Work out the finished part from the listing and answer in its coordinate system (mm). Give positions to 0.01 mm unless a question says otherwise; leave off trailing zeros. Loops run counter-clockwise (first coordinate to the right, second up) from the corner with the lowest first, then second, coordinate; pieces in that order, holes last. Notation, with made-up numbers: M 6.25,-1.75 L 12.25,-1.75 A24 cw 12.25,35.25 Z; hole C 80.5,24.5 d2. An arc over 180 degrees is marked long. Write item = value, one per line. Start each with the question number.
1. Section A-A on z = 1.85 is taken. Give the number of separate pieces and of enclosed holes in the cut face, plus the area to 3 significant figures.
2. Section C-C on y = 202.5 is taken. Determine the outline of the cut face in (x, z), plus the area to 4 significant figures.
3. Consider L1, parallel to Y at x = 146.5, z = 2.75; L2, parallel to X at y = 201, z = 3.15; L3, parallel to Y at x = 185, z = 5.05. Determine where each line is inside the solid, lowest interval first. Write a range as [from, to].
4. Section B-B on y = 85 is taken. Determine the outline of the cut face in (x, z), plus the area to 3 significant figures.
5. Flat-ended cylindrical pins translate along their axes: pin 1 Ø3 at (y, z) = (186, 4) entering from -X; pin 2 Ø1.6 at (y, z) = (170, 4) entering from +X. Find the tip coordinate at first contact, or state that the pin passes through.
6. The mould has two halves that part along X. Classify faces 1 (the face through (105, 164, 5.5)), 2 (the face through (64.105, 184.197, 2.788)): released by +X, released by -X, zero draft, split by the parting line, or undercut.
Autodesk Inventor part; units mm, degrees
ref_plane "YZ Plane" through (0, 0, 0) normal (1, 0, 0) x (0, 1, 0)
ref_plane "XZ Plane" through (0, 0, 0) normal (0, 1, 0) x (-1, 0, 0)
ref_plane "XY Plane" through (0, 0, 0) normal (0, 0, 1) x (1, 0, 0)
sketch "Sketch1" plane through (0, 0, 0) normal (0, 0, 1) x (1, 0, 0)
  line L0 (0, 0) -> (106.5, 0)
  line L1 (106.5, 0) -> (106.5, 232.6) construction
  line L2 (106.5, 232.6) -> (0, 232.6)
  line L3 (0, 232.6) -> (0, 0)
  line L4 (213, 0) -> (106.5, 0)
  line L5 (106.5, 232.6) -> (213, 232.6)
  line L6 (213, 232.6) -> (213, 0)
  line L7 (5.5, 100) -> (5.5, 232.599)
  line L8 (5.5, 232.599) -> (0, 232.599)
  line L9 (0, 232.599) -> (0, 100)
  line L10 (0, 100) -> (5.5, 100)
  line L11 (5.5, 100) -> (0, 232.599) construction
  line L12 (5.5, 232.599) -> (0, 100) construction
  line L13 (31, 100) -> (31, 232.599)
  line L14 (31, 232.599) -> (25.5, 232.599)
  line L15 (25.5, 232.599) -> (25.5, 100)
  line L16 (25.5, 100) -> (31, 100)
  line L17 (31, 100) -> (25.5, 232.599) construction
  line L18 (31, 232.599) -> (25.5, 100) construction
  line L19 (96.5, 100) -> (96.5, 232.599)
  line L20 (96.5, 232.599) -> (91.5, 232.599)
  line L21 (91.5, 232.599) -> (91.5, 100)
  line L22 (91.5, 100) -> (96.5, 100)
  line L23 (96.5, 100) -> (91.5, 232.599) construction
  line L24 (96.5, 232.599) -> (91.5, 100) construction
  line L25 (207.5, 100) -> (207.5, 232.599)
  line L26 (207.5, 232.599) -> (213, 232.599)
  line L27 (213, 232.599) -> (213, 100)
  line L28 (213, 100) -> (207.5, 100)
  line L29 (207.5, 100) -> (213, 232.599) construction
  line L30 (207.5, 232.599) -> (213, 100) construction
  line L31 (182, 100) -> (182, 232.599)
  line L32 (182, 232.599) -> (187.5, 232.599)
  line L33 (187.5, 232.599) -> (187.5, 100)
  line L34 (187.5, 100) -> (182, 100)
  line L35 (182, 100) -> (187.5, 232.599) construction
  line L36 (182, 232.599) -> (187.5, 100) construction
  line L37 (116.5, 100) -> (116.5, 232.599)
  line L38 (116.5, 232.599) -> (121.5, 232.599)
  line L39 (121.5, 232.599) -> (121.5, 100)
  line L40 (121.5, 100) -> (116.5, 100)
  line L41 (116.5, 100) -> (121.5, 232.599) construction
  line L42 (116.5, 232.599) -> (121.5, 100) construction
  line L43 (2.75, 166.2995) -> (94, 166.2995) construction
  point P0 (28.25, 166.2995)
  point P1 (210.25, 166.2995)
  point P2 (184.75, 166.2995)
  point P3 (119, 166.2995)
  point P4 (0, 100)
  point P5 (213, 100)
  point P6 (0, 232.599)
  dimension "d0" = 232.6
  dimension "d1" = 106.5
  dimension "d4" = 5.5
  dimension "d6" = 5.5
  dimension "d8" = 5
  dimension "d10" = 10
  dimension "d11" = 20
  dimension "d12" = 0
  dimension "d19" = 100
  dimension "d20" = 0.001
extrude "Extrusion1" add sketch "Sketch1" along normal blind 5.5 contours L3 L10 L7 L2 L15 L16 L13 L21 L22 L19 L5 L37 L40 L39 L31 L34 L33 L25 L28 L6 L4 L0
ref_plane "Work Plane3" through (61.25, 100, 0) normal (1, 0, 0) x (0, 0, -1)
sketch "Sketch2" plane through (0, 0, 5.5) normal (0, 0, 1) x (1, 0, 0)
  line L0 (0, 232.6) -> (213, 232.6)
  line L1 (213, 232.6) -> (213, 322.6)
  line L2 (213, 322.6) -> (0, 322.6)
  line L3 (0, 322.6) -> (0, 232.6)
  line L4 (213, 232.599) -> (213, 232.6)
  point P0 (0, 0)
  dimension "d15" = 90
extrude "Extrusion2" add sketch "Sketch2" against normal blind 5.5
sketch "Sketch3" plane through (0, 0, 5.5) normal (0, 0, 1) x (1, 0, 0)
  line L0 (213, 322.6) -> (0, 322.6) construction
  line L1 (31, 232.599) -> (31, 100) construction
  line L2 (91.5, 100) -> (91.5, 232.599) construction
  line L3 (121.5, 232.599) -> (121.5, 100) construction
  line L4 (31, 166.2995) -> (91.5, 166.2995) construction
  line L5 (91.5, 166.2995) -> (121.5, 166.2995) construction
  line L6 (106.5, 166.2995) -> (106.5, 322.6) construction
  circle A0 centre (66.5, 182) radius 3.25
  circle A1 centre (66.5, 85) radius 3.25
  circle A2 centre (146.5, 182) radius 3.25
  circle A3 centre (146.5, 85) radius 3.25
  line L7 (66.5, 85) -> (66.5, 182) construction
  line L8 (0, 0) -> (213, 0)
  dimension "d21" = 6.5
  dimension "d23" = 97
  dimension "d28" = 40
  dimension "d29" = 85
extrude "Extrusion3" cut sketch "Sketch3" against normal blind 10
ref_plane "Work Plane4" through (106.5, 100, 0) normal (1, 0, 0) x (0, 0, -1)
equation "\"d0\" = sidewallL + Uthick"
equation "\"d10\" = 0.5 * midbottomw"
equation "\"d11\" = lrbottomw"
equation "\"d19\" = Uthick"
equation "\"d15\" = wireL"
equation "\"d28\" = 0.5 * marshdistance"
equation "\"thick\" = 0.5"
equation "\"lrlr\" = 19"
equation "\"lrmid\" = 19.9"
equation "\"lrdepth\" = 3.3"
equation "\"mlr\" = 16.6"
equation "\"mmid\" = 24.7"
equation "\"mdepth\" = 4.5"
equation "\"lrltotal\" = 126.6"
equation "\"mltotal\" = 126.6"
equation "\"lrbetween\" = 52.1"
equation "\"mbetween\" = 49.5"
equation "\"toler\" = 1"
equation "\"lrbottomw\" = 20"
equation "\"tight\" = 0.08"
equation "\"stuckw\" = 6"
equation "\"sidewallL\" = 132.6"
equation "\"heaterH\" = 117.3"
equation "\"Uthick\" = 100"
equation "\"stickL\" = 3.5"
equation "\"wireH\" = 25"
equation "\"wireL\" = 90"
properties part number "deepest_layer"
Verdict:
q1.separate_pieces = 1
q1.enclosed_holes = 8
q1.area = 64,300 mm2
q2.outline = M 5.5,0 L 25.5,0 L 25.5,5.5 L 5.5,5.5 Z; M 31,0 L 91.5,0 L 91.5,5.5 L 31,5.5 Z; M 96.5,0 L 116.5,0 L 116.5,5.5 L 96.5,5.5 Z; M 121.5,0 L 182,0 L 182,5.5 L 121.5,5.5 Z; M 187.5,0 L 207.5,0 L 207.5,5.5 L 187.5,5.5 Z
q2.area = 995.5 mm2
q3.L1 = [0, 81.75], [88.25, 178.75], [185.25, 322.6]
q3.L2 = [5.5, 25.5], [31, 91.5], [96.5, 116.5], [121.5, 182], [187.5, 207.5]
q3.L3 = [0, 100], [232.6, 322.6]
q4.outline = M 0,0 L 63.25,0 L 63.25,5.5 L 0,5.5 Z; M 69.75,0 L 143.25,0 L 143.25,5.5 L 69.75,5.5 Z; M 149.75,0 L 213,0 L 213,5.5 L 149.75,5.5 Z
q4.area = 1,100 mm2
q5.pin_1 = 5.5
q5.pin_2 = 207.5
q6.face_1 = zero draft
q6.face_2 = undercut
